Geometry: final body of the model. Coordinates: model frame, mm. A direction names the side the tool comes from. Coordinates: 2 decimals unless noted, no trailing zeros. Put each result on its own line as item: value. Start each with the question number.
1) Reachability of faces 4 (the flat face through (7.938, 5, 2)), 5 (the flat face through (29, 0, 2)), 6 (the flat face through (-139.7, -47, 2)), 7 (the flat face through (22, 9.652, 2)) from +Z, -Z, +X, -X, +Y, -Y: full face, straight path, thin tool, end or side. Return the list, or none.
2) Section A-A on z = 1.95. Count the separate pieces of the cut face and the enclosed holes in it, and give its area (3 significant figures).
3) Draft query along X for faces 1 (the flat face through (20.638, 5, 2)), 2 (the cylindrical face through (-137.41, -37.1, 1.57)), 3 (the flat face through (-54, -17, 3.175)). Return one class per face: +X half, -X half, draft (parallel to the pull), parting line (faces both ways), or undercut.
4) Contact query for flat-ended pins moving along their axis: pin 1 Ø1.4 at (y, z) = (8, 1) entering from -X; pin 2 Ø1.6 at (x, z) = (9.5, 1) entering from -Y; pin 3 Ø1.5 at (x, z) = (-3, 0.5) entering from -Y. Output: stop coordinate, or through.
5) Material intervals for line 1 along X through (y, z) = (9, 1.8) (3 decimals); line 2 along Y through (x, z) = (4, 2.6) (3 decimals); line 3 along Y through (x, z) = (-119, 1.5), sorted ascending. Write a range as from..to.
```python
from build123d import *

# Parameters (mm, degrees)
SKETCH1_R           = 1.016
BOSS_EXTRUDE1_DEPTH = 3.175


with BuildPart() as part:
    # Sketch1 → Boss-Extrude1 (new body)
    with BuildSketch(Plane.XY):
        with BuildLine():
            Line((0, 0), (3.175, 0))
            Line((3.175, 0), (3.175, 3.175))
            Line((3.175, 3.175), (7.9375, 3.175))
            Line((7.9375, 3.175), (7.9375, 6.858))
            Line((7.9375, 6.858), (6.35, 6.858))
            Line((6.35, 6.858), (6.35, 9.652))
            Line((6.35, 9.652), (12.7, 9.652))
            Line((12.7, 9.652), (12.7, 6.858))
            Line((12.7, 6.858), (11.1125, 6.858))
            Line((11.1125, 6.858), (11.1125, 3.175))
            Line((11.1125, 3.175), (20.6375, 3.175))
            Line((20.6375, 3.175), (20.6375, 6.858))
            Line((20.6375, 6.858), (19.05, 6.858))
            Line((19.05, 6.858), (19.05, 9.652))
            Line((19.05, 9.652), (25.4, 9.652))
            Line((25.4, 9.652), (25.4, 6.858))
            Line((25.4, 6.858), (23.8125, 6.858))
            Line((23.8125, 6.858), (23.8125, 3.175))
            Line((23.8125, 3.175), (26.9875, 3.175))
            Line((26.9875, 3.175), (26.9875, 0))
            Line((26.9875, 0), (31.75, 0))
            Line((31.75, 0), (31.75, 15.875))
            Line((31.75, 15.875), (0, 15.875))
            add(Edge.make_bspline(
                [(-120.65, -34.925), (-86.994673616, -34.925), (-33.403901093, 15.875), (0, 15.875)],
                knots=[0, 0, 0, 0, 1, 1, 1, 1], degree=3))
            Line((-120.65, -34.925), (-132.08, -34.925))
            ThreePointArc((-132.08, -34.925), (-137.468153673, -37.156846327), (-139.7, -42.545))
            Line((-139.7, -42.545), (-139.7, -50.8))
            Line((-139.7, -50.8), (-128.27, -50.8))
            add(Edge.make_bspline(
                [(-128.27, -50.8), (-84.724287152, -50.8), (-32.997851809, 0), (0, 0)],
                knots=[0, 0, 0, 0, 1, 1, 1, 1], degree=3))
        make_face()
        with Locations((-131.7625, -39.0525)):
            Circle(SKETCH1_R, mode=Mode.SUBTRACT)
        with Locations((-131.7625, -46.6725)):
            Circle(SKETCH1_R, mode=Mode.SUBTRACT)
    extrude(amount=BOSS_EXTRUDE1_DEPTH)


solid = part.part
```
Answer block:
1. face 4: +Z, -Z, -Y
1. face 5: +Z, -Z, +X, -Y
1. face 6: +Z, -Z, -X, +Y, -Y
1. face 7: +Z, -Z
2. separate pieces: 1
2. enclosed holes: 2
2. area: 2,530 mm²
3. face 1: undercut
3. face 2: -X half
3. face 3: draft
4. pin 1: stops at x = -29.57
4. pin 2: stops at y = 9.65
4. pin 3: stops at y = -0.2
5. line 1: x = -25.875..6.35, 12.7..19.05, 25.4..31.75
5. line 2: y = 3.175..15.875
5. line 3: y = -50.09..-34.89
